Could you check a few things on this drawing? It's one solid part, dimensions in mm from its lowest x, y, z. A direction names the side the tool comes from. Round coordinates to 2 decimals unless told otherwise and drop trailing zeros. Write each loop counter-clockwise with the first axis right and the second up, starting at its lowest first coordinate (ties: lowest second). Pieces come first, ordered by that corner, then holes. Notation, with made-up numbers: (-7, -13) -> (51, -13) arc R23 ccw to (51, -5) -> close; hole circle Ø6 at (17, 87). An arc over 180 degrees is marked (long way). Put each result on its own line as item: value. Start each with the question number.
1) I want a section at D-D, the plane z = 8.75. List the corners of the cut face in (x, y) for me, then the cut area to 3 significant figures.
2) Will these pins go through, and if not, where does the flat tip stop? P1, Ø1.9, axis at y = 1, z = 17, coming from the +X side; P2, Ø1, axis at x = 2, y = 3.5, coming from the -Z side; P3, Ø1.2, axis at y = 1.5, z = 12.5, coming from the +X side; P4, Ø1.8, axis at y = 2.5, z = 20.5, coming from the +X side (1 decimal).
3) I want a section at C-C, the plane z = 20.5. List the corners of the cut face in (x, y) for me (1 decimal).
4) Which directions (+Z, -Z, +X, -X, +Y, -Y) give clear straight access to the entire face, cutting with the end or side of a thin tool? Please do the marked faces 1, 2 and 3.
5) If I drill on line 1 along X through (y, z) = (3.25, 12.25); line 2 along X through (y, z) = (0.4, 14.75); line 3 along Z through (x, y) = (3.95, 2.35), over which ranges is the centre line in solid material (lowest first)? Write a range as [from, to].
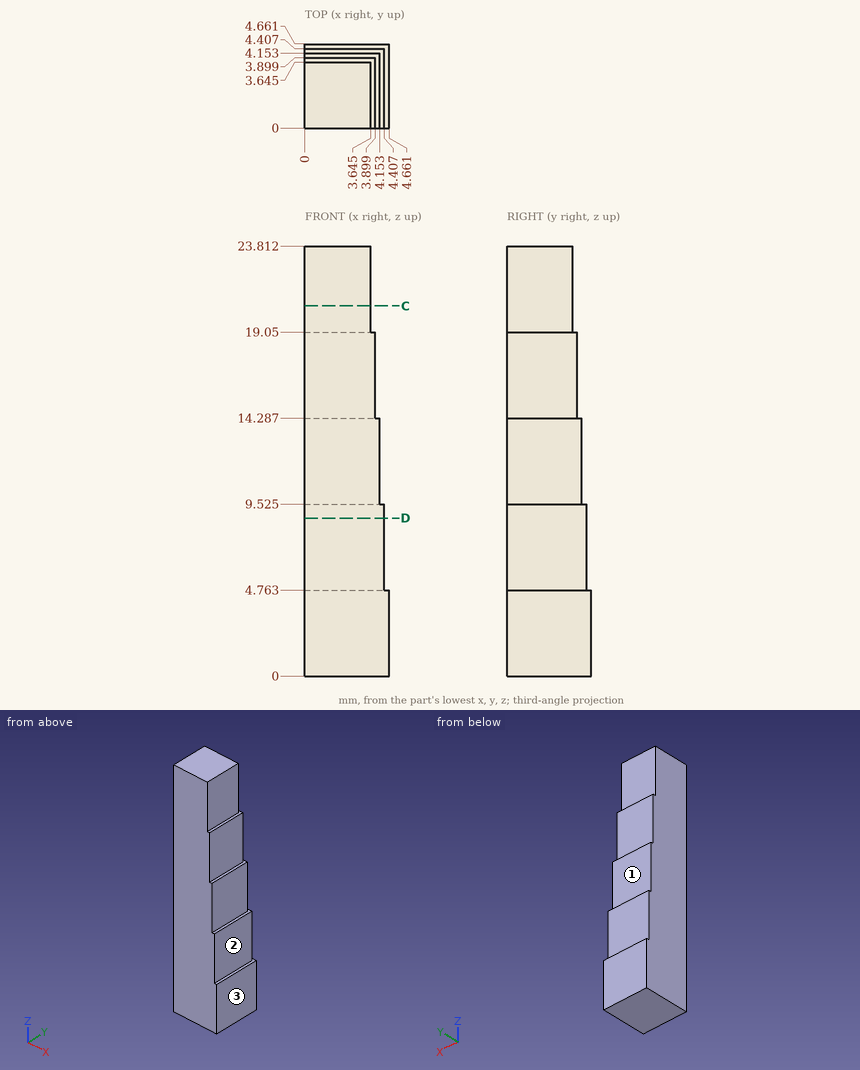
Findings:
1. outline: (0, 0) -> (4.41, 0) -> (4.41, 4.41) -> (0, 4.41) -> close
1. area: 19.4 mm2
2. P1: stops at x = 3.9
2. P2: stops at z = 0
2. P3: stops at x = 4.15
2. P4: stops at x = 3.6
3. outline: (0, 0) -> (3.6, 0) -> (3.6, 3.6) -> (0, 3.6) -> close
4. face 1: +Z, +X, -X, +Y
4. face 2: +Z, +X, +Y, -Y
4. face 3: +Z, -Z, +X, +Y, -Y
5. line 1: x = [0, 4.15]
5. line 2: x = [0, 3.9]
5. line 3: z = [0, 14.29]
